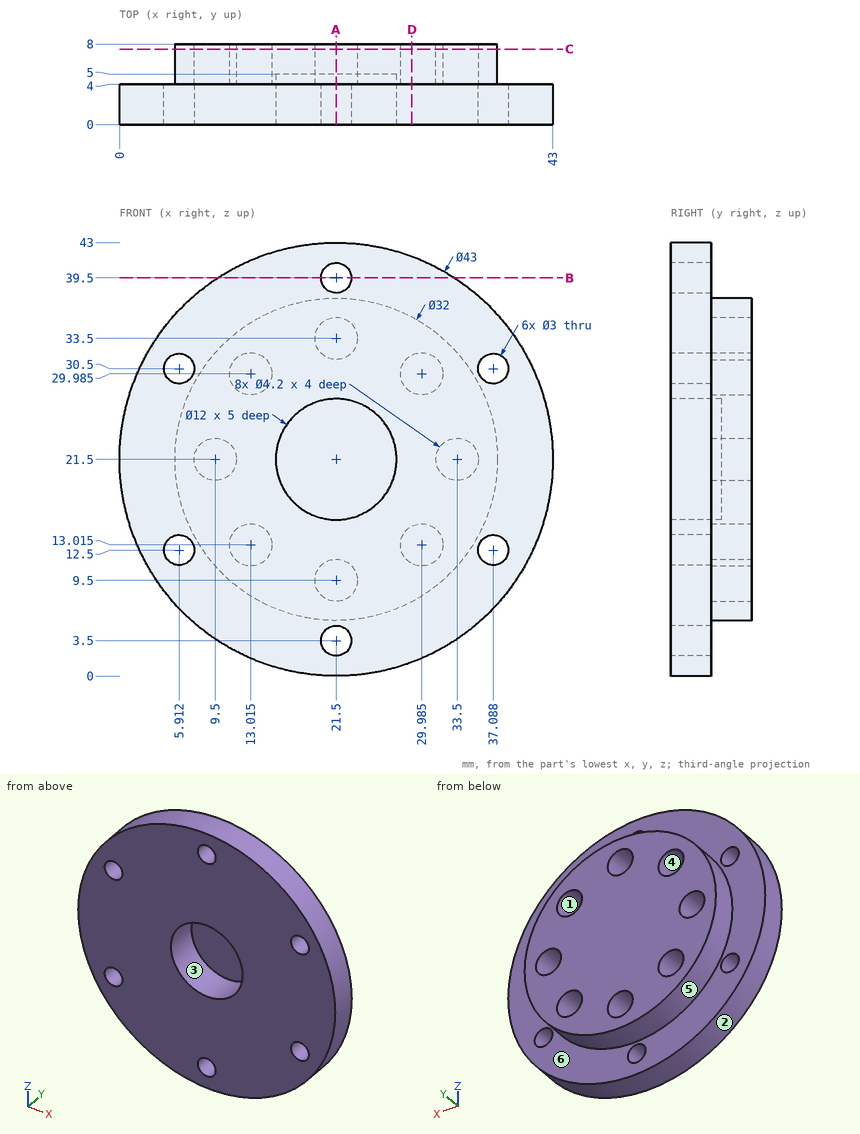
Job drawing, mm, ordinate dimensions from the low corner. One solid piece. A direction names the side the tool comes from. Give positions to 0.01 mm unless a question says otherwise; leave off trailing zeros. Write each loop counter-clockwise with the first axis right and the second up, starting at its lowest first coordinate (ties: lowest second). Pieces come first, ordered by that corner, then holes. Notation, with made-up numbers: M 65.5,-40 L 122.5,-40 A13 cw 122.5,-27 Z; hole C 81,45 d1. An arc over 180 degrees is marked long. One line per item, written item: value. Start each with the question number.
Q1. Saw through at B-B, the plane z = 39.5. Write the cut outline in (x, y).
Q2. Probe probe 1 along Z at (x, y) = (21.5, 7); probe 2 along Z at (x, y) = (21.5, 2.1); probe 3 along Z at (x, y) = (21.5, 4.9). List the from-to ranges inside material, lowest first. Write a range as [from, to].
Q3. Drop flat-ended pins along their axis: pin 1 Ø2.5 at (x, z) = (21.5, 3.5) entering from +Y; pin 2 Ø1 at (y, z) = (2.5, 12.5) entering from +X; pin 3 Ø8 at (x, z) = (6, 8.5) entering from +Y. Give the stop position or say it passes through.
Q4. Saw through at D-D, the plane x = 29. Write the cut outline in (y, z).
Q5. Saw through at C-C, the plane y = 7.5. State how many separate pieces and enclosed holes the cut face has.
Q6. Two-plate mould, pull along Z, no slides. Class the marked faces 4, 5 and 6: +Z half, -Z half, draft (parallel to the pull), parting line (faces both ways), or undercut.
Q7. Saw through at A-A, the plane x = 21.5. Write the cut outline in (y, z).
Q8. 3-axis set-ups, long thin cutter, end or side, ignore diameter. For the marked faces 1, 2 and 3: which of +Z, -Z, +X, -X, +Y, -Y reach the whole face in a straight line?
Output values:
1. outline: M 9.74,0 L 20,0 L 20,4 L 9.74,4 Z; M 23,0 L 33.26,0 L 33.26,4 L 23,4 Z
2. probe 1: z = [5.5, 7.4], [11.6, 31.4], [35.6, 37.5]
2. probe 2: z = [0, 2], [5, 15.5], [27.5, 38], [41, 43]
2. probe 3: z = [5.5, 7.4], [11.6, 15.5], [27.5, 31.4], [35.6, 37.5]
3. pin 1: passes through
3. pin 2: stops at x = 41.25
3. pin 3: stops at y = 4
4. outline: M 0,1.35 L 4,1.35 L 4,7.37 L 8,7.37 L 8,11.16 L 4,11.16 L 4,14.87 L 8,14.87 L 8,28.13 L 4,28.13 L 4,31.84 L 8,31.84 L 8,35.63 L 4,35.63 L 4,41.65 L 0,41.65 Z
5. separate pieces: 1
5. enclosed holes: 8
6. face 4: undercut
6. face 5: parting line
6. face 6: draft
7. outline: M 0,0 L 4,0 L 4,2 L 0,2 Z; M 0,5 L 4,5 L 4,5.5 L 8,5.5 L 8,7.4 L 4,7.4 L 4,11.6 L 8,11.6 L 8,31.4 L 4,31.4 L 4,35.6 L 8,35.6 L 8,37.5 L 4,37.5 L 4,38 L 0,38 L 0,27.5 L 5,27.5 L 5,15.5 L 0,15.5 Z; M 0,41 L 4,41 L 4,43 L 0,43 Z
8. face 1: +Y
8. face 2: +Y, -Y
8. face 3: -Y
